Source: CAD feature listing. Evaluate the final solid. Frame: model axes, mm. Give positions to 0.01 mm unless a question says otherwise; leave off trailing zeros. Write each loop counter-clockwise with the first axis right and the second up, starting at its lowest first coordinate (ties: lowest second). Pieces come first, ordered by that corner, then holes. Notation, with made-up numbers: (61.25, -11.75) - (119.25, -11.75) arc R27 cw to (119.25, 24.25) - close; hole circle Ø6 at (37, -32.75). An arc over 180 degrees is marked (long way). Answer as a JSON object with one key per item and string values. Group by question number.
from build123d import *

# Parameters (mm, degrees)
ESQUISSE1_W                               = 13.5
ESQUISSE1_H                               = 8
BOSS_EXTRU_1_DEPTH                        = 5
TROU_POUR_TARAUDAGE_POUR_TROU_TARAUD_M2_D = 1.6
KERNLOCH_F_R_M3_GEWINDE1_D                = 2.5
KERNLOCH_F_R_M3_GEWINDE1_DEPTH            = 5
KERNLOCH_F_R_M3_GEWINDE1_TIP              = 0.751075774


with BuildPart() as part:
    # Esquisse1 → Boss.-Extru.1 (new body)
    with BuildSketch(Plane.XY):
        with Locations((6.75, 4)):
            Rectangle(ESQUISSE1_W, ESQUISSE1_H)
    extrude(amount=BOSS_EXTRU_1_DEPTH)

    # Trou pour taraudage pour trou taraudé M21 (through all)
    with Locations(Plane.ZY):
        with Locations((2.5, 6), (2.5, 1.5)):
            Hole(TROU_POUR_TARAUDAGE_POUR_TROU_TARAUD_M2_D / 2)

    # Kernloch für M3 Gewinde1
    with Locations(Plane(origin=(0, 0, 0), x_dir=(-1, 0, 0), z_dir=(0, 0, -1))):
        with Locations((-6.75, 5.5)):
            Hole(KERNLOCH_F_R_M3_GEWINDE1_D / 2, depth=KERNLOCH_F_R_M3_GEWINDE1_DEPTH)
            with Locations((0, 0, -(KERNLOCH_F_R_M3_GEWINDE1_DEPTH + KERNLOCH_F_R_M3_GEWINDE1_TIP / 2))):  # 118° drill point
                Cone(0, KERNLOCH_F_R_M3_GEWINDE1_D / 2, KERNLOCH_F_R_M3_GEWINDE1_TIP, mode=Mode.SUBTRACT)


solid = part.part
Q1. Section C-C on y = 1.5. Return the cut outline in (x, z), then the cut area to 3 significant figures.
Q2. Section B-B on z = 3.85. Return the cut outline in (x, y), then the cut area to 3 significant figures.
Q3. Draft query along X for faces 1 (the cylindrical face through (7.327, 4.391, 2.535)), 2 (the flat face through (0, 4, 2)), 3 (the flat face through (7, 0, 2)). Return one class per face: released by +X, released by -X, zero draft, split by the parting line, or undercut.
Q4. Ray query, probe 1 along Y at (x, z) = (9, 2.5); probe 2 along Y at (x, z) = (6.75, 1.25); probe 3 along Y at (x, z) = (4.5, 3.1). Return the intervals inside material, ascending. Write a range as [from, to].
Q5. Section D-D on y = 5.5. Return the cut outline in (x, z).
Q6. Section A-A on x = 6.25. Return the cut outline in (y, z).
Taken from the geometry:
{
 "1": {"outline": "(0, 0) - (13.5, 0) - (13.5, 1.7) - (0, 1.7) - close; (0, 3.3) - (13.5, 3.3) - (13.5, 5) - (0, 5) - close", "area": "45.9 mm²"},
 "2": {"outline": "(0, 0) - (13.5, 0) - (13.5, 8) - (0, 8) - close; hole circle Ø2.5 at (6.75, 5.5)", "area": "103 mm²"},
 "3": {"face 1": "undercut", "face 2": "released by -X", "face 3": "zero draft"},
 "4": {"probe 1": "y = [0, 0.7], [2.3, 5.2], [6.8, 8]", "probe 2": "y = [0, 4.25], [6.75, 8]", "probe 3": "y = [0, 0.97], [2.03, 5.47], [6.53, 8]"},
 "5": {"outline": "(0, 0) - (5.5, 0) - (5.5, 1.88) - (0, 1.88) - close; (0, 3.12) - (5.5, 3.12) - (5.5, 5) - (0, 5) - close; (8, 0) - (13.5, 0) - (13.5, 1.88) - (8, 1.88) - close; (8, 3.12) - (13.5, 3.12) - (13.5, 5) - (8, 5) - close"},
 "6": {"outline": "(0, 0) - (4.35, 0) - (4.35, 5) - (0, 5) - close; (6.65, 0) - (8, 0) - (8, 5) - (6.65, 5) - (6.65, 2.97) arc R0.8 cw to (6.65, 2.03) - close; hole circle Ø1.6 at (1.5, 2.5)"}
}
